Build history of the part. All positions in model axes, mm. Round coordinates to 2 decimals unless told otherwise and drop trailing zeros. Order: outer loops, then holes, each group sorted by start corner. A loop starts at its lowest first (then second) coordinate and runs counter-clockwise, first axis right, second up. Notation, with made-up numbers: (-22, 51) -> (-14, 51) arc R23 cw to (-14, 66) -> close; hole circle Ø2 at (0, 86). An arc over 180 degrees is marked (long way). Answer as a JSON object with one key per item and string values.
from build123d import *

# Parameters (mm, degrees)
SKETCH1_R             = 6.5
SKETCH1_R_2           = 11.5
BOSS_EXTRUDE1_DEPTH   = 10
CHAMFER1_SIZE         = 2
M4X0_7_TAPPED_HOLE1_D = 3.3
M4X0_7_TAPPED_HOLE2_D = 3.3
CIRPATTERN1_COUNT     = 3
MIRROR1_COPY_1_D      = 3.3
MIRROR1_COPY_2_D      = 3.3


with BuildPart() as part:
    # Sketch1 → Boss-Extrude1 (new body)
    with BuildSketch(Plane(origin=(0, 0, 0), x_dir=(1, 0, 0), z_dir=(0, 1, 0))):
        Polygon((-105, -35), (-20, 75), (20, 75), (105, -35), (105, -75), (65, -75), (-65, -75), (-105, -75), align=None)
        with Locations(Location((-30, 0, 0), (0, 0, 270))):
            Circle(SKETCH1_R, mode=Mode.SUBTRACT)
        with Locations(Location((30, 0, 0), (0, 0, 270))):
            Circle(SKETCH1_R, mode=Mode.SUBTRACT)
        with Locations(Location((0, 55, 0), (0, 0, 270))):
            Circle(SKETCH1_R_2, mode=Mode.SUBTRACT)
        with Locations(Location((85, -55, 0), (0, 0, 270))):
            Circle(SKETCH1_R_2, mode=Mode.SUBTRACT)
        with Locations(Location((-85, -55, 0), (0, 0, 270))):
            Circle(SKETCH1_R_2, mode=Mode.SUBTRACT)
    extrude(amount=BOSS_EXTRUDE1_DEPTH)

    # Chamfer1
    chamfer1_edges = [part.edges().sort_by_distance(p)[0] for p in [
        (105, 5, 75),
        (-105, 5, 75),
    ]]
    chamfer(chamfer1_edges, length=CHAMFER1_SIZE)

    # M4x0.7 Tapped Hole1 (through all)
    with Locations(Plane(origin=(-96.313708499, 10, 43.686291501), x_dir=(0, 0, 1), z_dir=(0, 1, 0))):
        with Locations((0, 0), (0, 22.627416998), (22.627416998, 22.627416998), (22.627416998, 0), (-87.372583002, 85), (-110, 85)):
            m4x0_7_tapped_hole1 = Hole(M4X0_7_TAPPED_HOLE1_D / 2)

    # M4x0.7 Tapped Hole2 (through all)
    with Locations(Plane(origin=(-12, 10, 0), x_dir=(0, 0, 1), z_dir=(0, 1, 0))):
        with Locations((0, 0)):
            m4x0_7_tapped_hole2 = Hole(M4X0_7_TAPPED_HOLE2_D / 2)

    # CirPattern1: M4x0.7 Tapped Hole2 ×3 about axis
    cirpattern1_axis = Axis((-30, 0, 0), (0, 1, 0))
    for i in range(1, CIRPATTERN1_COUNT):
        add(m4x0_7_tapped_hole2.rotate(cirpattern1_axis, i * 360 / CIRPATTERN1_COUNT), mode=Mode.SUBTRACT)

    # Mirror1: M4x0.7 Tapped Hole1, M4x0.7 Tapped Hole2 across plane
    add(m4x0_7_tapped_hole1.mirror(Plane(origin=(0, 0, 0), x_dir=(0, 0, 1), z_dir=(1, 0, 0))), mode=Mode.SUBTRACT)
    add(m4x0_7_tapped_hole2.mirror(Plane(origin=(0, 0, 0), x_dir=(0, 0, 1), z_dir=(1, 0, 0))), mode=Mode.SUBTRACT)

    # Mirror1 copy 1 (through all)
    with Locations(Plane(origin=(39, 10, -15.588457268), x_dir=(-0.8660254037844387, 0, -0.4999999999999998), z_dir=(0, 1, 0))):
        with Locations((0, 0)):
            Hole(MIRROR1_COPY_1_D / 2)

    # Mirror1 copy 2 (through all)
    with Locations(Plane(origin=(39, 10, 15.588457268), x_dir=(0.8660254037844384, 0, -0.5000000000000004), z_dir=(0, 1, 0))):
        with Locations((0, 0)):
            Hole(MIRROR1_COPY_2_D / 2)


solid = part.part
1) Cut at D-D, the plane z = -30.5. Give the cut face in (x, y), plus the area to 3 significant figures.
Checked values:
{"outline": "(-54.39, 0) -> (54.39, 0) -> (54.39, 10) -> (-54.39, 10) -> close", "area": "1,090 mm²"}
2) Cut at C-C, the plane z = -55. Give the cut face in (x, y).
Checked values:
{"outline": "(-35.45, 0) -> (-11.5, 0) -> (-11.5, 10) -> (-35.45, 10) -> close; (11.5, 0) -> (35.45, 0) -> (35.45, 10) -> (11.5, 10) -> close"}
3) Pull direction X, two halves, no side cores. Call faces 1 (the face through (1, 10, 16)), 2 (the face through (-105, 5, 54)), 3 (the face through (36.445, 4.93, -0.846)), 4 (the face through (3.45, 4.93, -44.03)): pulls with the +X half, pulls with the -X half, needs draft (parallel to the pull), parting line crosses it, or undercut.
Checked values:
{"face 1": "needs draft", "face 2": "pulls with the -X half", "face 3": "undercut", "face 4": "undercut"}
4) Cut at A-A, the plane x = 30. Give the cut face in (y, z), plus the area to 3 significant figures.
Checked values:
{"outline": "(0, -62.06) -> (10, -62.06) -> (10, -6.5) -> (0, -6.5) -> close; (0, 6.5) -> (10, 6.5) -> (10, 75) -> (0, 75) -> close", "area": "1,240 mm²"}
5) Cut at B-B, the plane y = 5.5. Count the separate pieces of the cut face and the enclosed holes in it, plus the area to 3 significant figures.
Checked values:
{"separate pieces": "1", "enclosed holes": "23", "area": "20,500 mm²"}
6) Probe L1, parallel to X at y = 2.5, z = 62; L2, parallel to X at y = 5.25, z = -17; L3, parallel to X at y = 4, z = 0. List the from-to ranges inside material, lowest first. Write a range as from..to.
Checked values:
{"L1": "x = -105..-94.12, -75.88..75.88, 94.12..105", "L2": "x = -64.82..-39.85, -38.15..38.15, 39.85..64.82", "L3": "x = -77.95..-36.5, -23.5..-13.65, -10.35..10.35, 13.65..23.5, 36.5..77.95"}
7) Flat gauge pins, fed straight in: pin 1 Ø5 at (y, z) = (9, 4) entering from -X; pin 2 Ø6 at (x, y) = (-74, 7.5) entering from -Z. Where does each tip first touch, or does it go through?
Checked values:
{"pin 1": "stops at x = -82.98", "pin 2": "stops at z = -9"}
